```python
from build123d import *

# Parameters (mm, degrees)
F_9_0_9_DIAMETER_HOLE1_D = 9
CIRPATTERN1_COUNT        = 6
CHAMFER1_SIZE            = 1
EXTRUDE1_DEPTH           = 58.933971161


with BuildPart() as part:
    # Sketch1 → Revolve1 (revolve)
    with BuildSketch(Plane(origin=(0, 0, 0), x_dir=(0, 0, -1), z_dir=(1, 0, 0)), mode=Mode.PRIVATE) as revolve1_sk:
        Polygon((0, 18), (8.5, 18), (8.5, 19), (10.1, 19), (10.1, 18), (12.5038, 18), (12.5038, 23.5), (7.5, 23.5), (7.5, 40), (0, 40), align=None)
    revolve(revolve1_sk.sketch.rotate(Axis((0, 0, -13.627513848), (0, 0, 1)), 90), axis=Axis((0, 0, -13.627513848), (0, 0, 1)))

    # Ø9.0 (9) Diameter Hole1 (through all)
    with Locations(Plane(origin=(0, 0, -7.5), x_dir=(-1, 0, 0), z_dir=(0, 0, -1))):
        with Locations((0, 29.25)):
            f_9_0_9_diameter_hole1 = Hole(F_9_0_9_DIAMETER_HOLE1_D / 2)

    # CirPattern1: Ø9.0 (9) Diameter Hole1 ×6 about axis
    cirpattern1_axis = Axis((0, 0, 0), (0, 0, 1))
    for i in range(1, CIRPATTERN1_COUNT):
        add(f_9_0_9_diameter_hole1.rotate(cirpattern1_axis, i * 360 / CIRPATTERN1_COUNT), mode=Mode.SUBTRACT)

    # Chamfer1
    chamfer1_edges = [part.edges().sort_by_distance(p)[0] for p in [
        (23.5, 0, -12.5038),
    ]]
    chamfer(chamfer1_edges, length=CHAMFER1_SIZE)

    # Sketch4 → Extrude1 (cut, through all)
    with BuildSketch(Plane.XY):
        with BuildLine():
            Line((-35, 19.364916731), (-35, -19.364916731))
            ThreePointArc((-35, -19.364916731), (-40, 0), (-35, 19.364916731))
        make_face()
        with BuildLine():
            Line((35, 19.364916731), (35, -19.364916731))
            ThreePointArc((35, -19.364916731), (40, 0), (35, 19.364916731))
        make_face()
    extrude(amount=-EXTRUDE1_DEPTH, mode=Mode.SUBTRACT)


solid = part.part
```
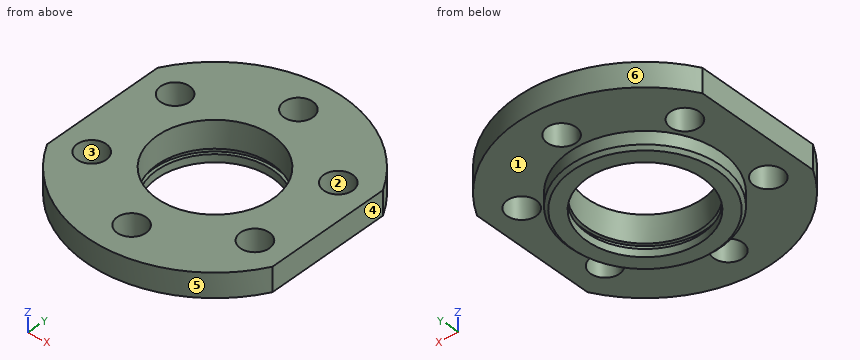
Design review of the part built by this model. Coordinates are the model's own, in mm. Face numbers are marked on the shaded views. A direction names the side the tool comes from. Coordinates: 2 decimals unless noted, no trailing zeros. Order: outer loops, then holes, each group sorted by start corner. A loop starts at its lowest first (then second) coordinate and runs counter-clockwise, first axis right, second up. Notation, with made-up numbers: M 53,-18.5 L 106,-18.5 A8 cw 106,-6.5 Z; hole C 44,23.25 d1. An arc over 180 degrees is marked long. Answer as a JSON object with one key per item and string values. Group by question number.
1) Tool access review of the marked faces 1 and 2: name each direction out of +Z, -Z, +X, -X, +Y, -Y from which nothing blocks a thin tool from reaching the whole face with its end or side.
2) Add section D-D, the plane y = -32. Write out the cut boundary in (x, z), then the cut area to 3 significant figures.
3) Add section C-C, the plane x = 24.5. Write out the cut boundary in (y, z).
4) Add section A-A, the plane x = 0. Count the separate pieces of the cut face and the enclosed holes in it, then the cut area to 3 significant figures.
5) Add section B-B, the plane y = 0. Write out the cut boundary in (x, z).
6) Mouldability with a two-part tool opening along Y and no side actions: class the marked faces 3, 4, 5 and 6 as pulls with the +Y half, pulls with the -Y half, needs draft (parallel to the pull), parting line crosses it, or undercut.
7) For pin 1 (1.5 mm diameter, centred on x = -5.5, z = -4, fed in from +Y); pin 2 (1 mm diameter, centred on x = -27.5, z = -3.5, fed in from -Y); pin 3 (12 mm diameter, centred on x = 13, y = -23.5, fed in from +Z); pin 4 (4 mm diameter, centred on y = 22, z = -6.5, fed in from -X), all flat-tipped, find the tip position at first contact; note any pin that passes through.
8) Wall thickness on L1, parallel to Y at x = 0, z = -1.25; L2, parallel to X at y = -13.5, z = -4.5; L3, parallel to Y at x = -24.5, z = -4.5: over which ranges is each line inside the solid? List them lowest first.
Computed values:
{
 "1": {"face 1": "-Z", "face 2": "+Z, -Z"},
 "2": {"outline": "M -24,-7.5 L -3.56,-7.5 L -3.56,0 L -24,0 Z; M 3.56,-7.5 L 24,-7.5 L 24,0 L 3.56,0 Z", "area": "307 mm^2"},
 "3": {"outline": "M -31.62,-7.5 L -19.05,-7.5 L -19.05,0 L -31.62,0 Z; M -10.2,-7.5 L 10.2,-7.5 L 10.2,0 L -10.2,0 Z; M 19.05,-7.5 L 31.62,-7.5 L 31.62,0 L 19.05,0 Z"},
 "4": {"separate pieces": "4", "enclosed holes": "0", "area": "246 mm^2"},
 "5": {"outline": "M -35,-7.5 L -23.5,-7.5 L -23.5,-11.5 L -22.5,-12.5 L -18,-12.5 L -18,-10.1 L -19,-10.1 L -19,-8.5 L -18,-8.5 L -18,0 L -35,0 Z; M 18,-12.5 L 22.5,-12.5 L 23.5,-11.5 L 23.5,-7.5 L 35,-7.5 L 35,0 L 18,0 L 18,-8.5 L 19,-8.5 L 19,-10.1 L 18,-10.1 Z"},
 "6": {"face 3": "undercut", "face 4": "needs draft", "face 5": "pulls with the -Y half", "face 6": "pulls with the +Y half"},
 "7": {"pin 1": "stops at y = 39.72", "pin 2": "stops at y = -29.51", "pin 3": "stops at z = 0", "pin 4": "stops at x = -34.64"},
 "8": {"L1": "y = -40 to -33.75, -24.75 to -18, 18 to 24.75, 33.75 to 40", "L2": "x = -35 to -29.69, -20.97 to -11.91, 11.91 to 20.97, 29.69 to 35", "L3": "y = -31.62 to -19.05, -10.2 to 10.2, 19.05 to 31.62"}
}
